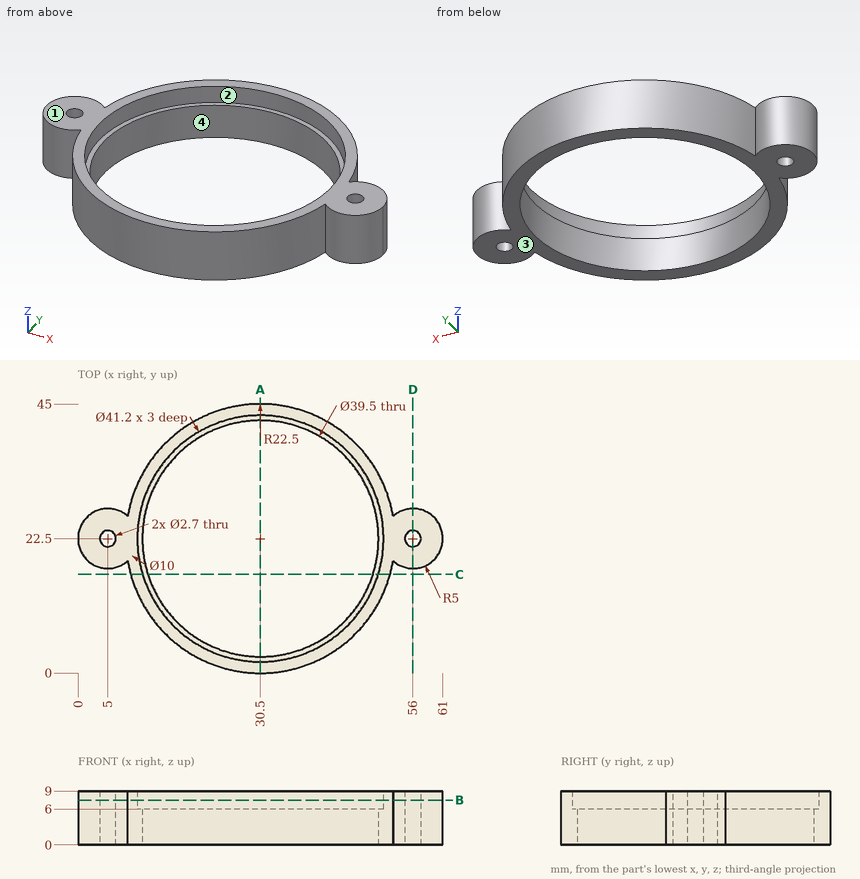
Design review of the part shown in the three views and the two pictorial views. Dimensions are in mm from the part's minimum x, y and z. A direction names the side the tool comes from. Give positions to 0.01 mm unless a question says otherwise; leave off trailing zeros. Write each loop counter-clockwise with the first axis right and the second up, starting at its lowest first coordinate (ties: lowest second). Pieces come first, ordered by that corner, then holes. Notation, with made-up numbers: M -9.75,-10.5 L 30.25,-10.5 A17 ccw 30.25,6.5 Z; hole C 1.25,32 d5. An arc over 180 degrees is marked long. Return JSON: item names as keys, results as strings. Group by question number.
Item 1: The part is to be moulded in two halves that separate along X. For the marked faces 3 and 4, say which applies: pulls with the +X half, pulls with the -X half, needs draft (parallel to the pull), parting line crosses it, or undercut.
Item 2: Clearance check with flat-ended pins moving along their axes: pin 1 Ø1.6 at (x, y) = (5, 22.5) entering from -Z; pin 2 Ø5 at (x, z) = (34, 3) entering from -Y; pin 3 Ø4 at (x, z) = (23, 3.5) entering from +Y; pin 4 Ø12 at (x, y) = (45, 22.5) entering from +Z. State where each tip first meets the part, or that it passes through.
Item 3: Take a section at A-A (x = 30.5). Give the boundary of the cut face in (y, z).
Item 4: Take a section at B-B (z = 7.5). Give the boundary of the cut face in (x, y), plus the area to 3 significant figures.
Item 5: Tool access review of the marked faces 1 and 2: name each direction out of +Z, -Z, +X, -X, +Y, -Y from which nothing blocks a thin tool from reaching the whole face with its end or side.
Item 6: Take a section at D-D (x = 56). Give the boundary of the cut face in (y, z).
Item 7: Wall thickness on line 1 along Y through (x, z) = (5, 3); line 2 along Y through (x, z) = (23, 2.25); line 3 along X through (y, z) = (31, 1.75): over which ranges is each line inside the solid? List them lowest first.
Item 8: Take a section at C-C (y = 16.5). Give the boundary of the cut face in (x, z).
Return value:
{
 "1": {"face 3": "needs draft", "face 4": "undercut"},
 "2": {"pin 1": "passes through", "pin 2": "stops at y = 0.02", "pin 3": "stops at y = 44.32", "pin 4": "stops at z = 6"},
 "3": {"outline": "M 0,0 L 2.75,0 L 2.75,6 L 1.9,6 L 1.9,9 L 0,9 Z; M 42.25,0 L 45,0 L 45,9 L 43.1,9 L 43.1,6 L 42.25,6 Z"},
 "4": {"outline": "M 8.31,18.76 A22.5 ccw 52.69,18.76 A5 ccw long 52.69,26.24 A22.5 ccw 8.31,26.24 A5 ccw long Z; hole C 5,22.5 d2.7; hole C 30.5,22.5 d41.2; hole C 56,22.5 d2.7", "area": "382 mm2"},
 "5": {"face 1": "+Z, +X, -X, +Y, -Y", "face 2": "+Z"},
 "6": {"outline": "M 17.5,0 L 21.15,0 L 21.15,9 L 17.5,9 Z; M 23.85,0 L 27.5,0 L 27.5,9 L 23.85,9 Z"},
 "7": {"line 1": "y = 17.5 to 21.15, 23.85 to 27.5", "line 2": "y = 1.29 to 4.23, 40.77 to 43.71", "line 3": "x = 9.67 to 12.67, 48.33 to 51.33"},
 "8": {"outline": "M 8.81,0 L 11.68,0 L 11.68,6 L 10.79,6 L 10.79,9 L 8.81,9 Z; M 49.32,0 L 52.19,0 L 52.19,9 L 50.21,9 L 50.21,6 L 49.32,6 Z"}
}
